For this review, take the finished solid that the model builds, in its own axes (mm). A direction names the side the tool comes from. Coordinates: 2 decimals unless noted, no trailing zeros. Write each loop counter-clockwise with the first axis right and the second up, starting at its lowest first coordinate (ties: lowest second). Pieces come first, ordered by that corner, then holes.
1) Mouldability with a two-part tool opening along Z and no side actions: class faces 1 (the face through (0, 15, -13.465)), 2 (the face through (-12.073, 24.775, -14.204)), 3 (the face through (0, 15, 13.465)), 4 (the face through (0, 16, 14.965)) as pulls with the +Z half, pulls with the -Z half, needs draft (parallel to the pull), parting line crosses it, or undercut.
2) For faces 5 (the face through (0, 1.5, 0)), 6 (the face through (0.338, 29.578, -14.226)), 7 (the face through (0, 0, 0)), list the 3-axis set-ups (+Z, -Z, +X, -X, +Y, -Y) from which the entire face can be reached by the end or side of a thin tool; tool diameter is ignored.
3) We need section B-B on x = 0. Write out the cut boundary in (y, z) (3 decimals).
4) Insertion check: P1, Ø1.5, axis at x = -2.5, z = -2.5, coming from the +Y side; P2, Ø7, axis at x = 0, y = 27, coming from the -Z side (3 decimals); P3, Ø1.9, axis at x = -7, y = 27, coming from the -Z side (3 decimals). Each pin has a flat end and moves straight along its axis. Give the tip position at first contact, or say it passes through.
5) To check wall thickness, follow line 1 along Z through (x, y) = (-12, 3.5) (3 decimals); line 2 along Y through (x, z) = (13, 8.25); line 3 along Y through (x, z) = (-7, -13.95). State the ranges of each line that lie inside material, in increasing order.
6) We need section C-C on x = -7. Write out the cut boundary in (y, z) (3 decimals).
7) We need section A-A on y = 4. Write out the cut boundary in (x, z) (3 decimals).
8) We need section D-D on y = 27. Write out the cut boundary in (x, z) (3 decimals), then the cut area to 3 significant figures.
Autodesk Inventor part; units mm, degrees
ref_plane "YZ Plane" through (0, 0, 0) normal (1, 0, 0) x (0, 1, 0)
ref_plane "XZ Plane" through (0, 0, 0) normal (0, 1, 0) x (-1, 0, 0)
ref_plane "XY Plane" through (0, 0, 0) normal (0, 0, 1) x (1, 0, 0)
sketch "Sketch1" plane through (0, 0, 0) normal (0, 1, 0) x (-1, 0, 0)
  line L0 (15, 14.965) -> (-15, 14.965)
  line L1 (-15, 14.965) -> (-15, -14.965)
  line L2 (-15, -14.965) -> (15, -14.965)
  line L3 (15, -14.965) -> (15, 14.965)
  point P0 (0, 0)
  dimension "d0" = 29.93
  dimension "d1" = 30
  dimension "d2" = 15
  dimension "d3" = 14.965
extrude "Plate1" add sketch "Sketch1" along normal blind 1.5
sketch "Sketch2" plane through (-15, 0, -13.465) normal (0, 0, -1) x (-1, 0, 0)
  line L0 (-30, 0) -> (0, 0)
  line L1 (0, 0) -> (0, 37)
  line L2 (0, 37) -> (-30, 37)
  line L3 (-30, 37) -> (-30, 0)
edge flange "Flange1" height 37 angle 90 thickness 1.5 bend radius 0.31 thickness toward (0, 0, -1) relief tear relief width 1.5 relief depth 0.75 corner gap 0.31 corner form 0 edges at (0, 1.5, -14.965) (0, 1.5, 14.965) wall of the first edge with corners at (15, 0, -13.465) (-15, 0, -13.465) (-15, 37, -13.465) (15, 37, -13.465)
bend "Bend1"
corner "Corner1"
sketch "Sketch3" plane through (-15, 37, 14.965) normal (0, 0, 1) x (1, 0, 0)
  line L0 (0, 0) -> (30, 0)
  line L1 (0, -35.19) -> (0, 0)
  circle A0 centre (15, -10) radius 10
  line L2 (0, -18.5) -> (30, -18.5)
  line L3 (30, -18.5) -> (30, -28.5)
  line L4 (30, -28.5) -> (0, -28.5)
  line L5 (0, -28.5) -> (0, -18.5)
  line L6 (30, -18.5) -> (24.0624, -5.7723)
  line L7 (0, -18.5) -> (5.9376, -5.7723)
  line L8 (0, 0) -> (30, 0)
  line L9 (30, 0) -> (30, -25)
  line L10 (30, -25) -> (0, -25)
  line L11 (0, -25) -> (0, 0)
  point P0 (15, -37)
  point P1 (15, 0)
  dimension "d15" = 10
  dimension "d16" = 0
  dimension "d17" = 20
  dimension "d18" = 8.5
  dimension "d19" = 0
  dimension "d20" = 30
  dimension "d21" = 10
  dimension "d22" = 25
extrude "Extrusion1" cut sketch "Sketch3" against normal blind 35 contours L0 A0 L7 L1 | L0 L9 L6 A0
sketch "Sketch4" plane through (15, 1.81, -14.965) normal (0, 0, -1) x (-1, 0, 0)
  arc A0 (24.0624, 29.4177) -> (5.9376, 29.4177) centre (15, 25.19) ccw
  circle A1 centre (15, 25.19) radius 2.6
  circle A2 centre (8, 25.19) radius 1.05
  circle A3 centre (22, 25.19) radius 1.05
  circle A4 centre (15, 32.19) radius 1.05
  circle A5 centre (15, 18.19) radius 1.05
  point P0 (15, -1.81)
  dimension "d25" = 5.2
  dimension "d26" = 0
  dimension "d27" = 7
  dimension "d28" = 2.1
  dimension "d29" = 7
  dimension "d30" = 0
  dimension "d31" = 2.1
  dimension "d32" = 0
  dimension "d33" = 7
  dimension "d34" = 2.1
  dimension "d35" = 7
  dimension "d36" = 0
  dimension "d37" = 2.1
extrude "Extrusion2" cut sketch "Sketch4" against normal blind 1.5
sketch "Sketch5" plane through (-15, 1.81, 14.965) normal (0, 0, 1) x (1, 0, 0)
  arc A0 (24.0624, 29.4177) -> (5.9376, 29.4177) centre (15, 25.19) ccw
  circle A1 centre (15, 25.19) radius 2.55
  point P0 (15, -1.81)
  dimension "d40" = 5.1
extrude "Extrusion3" cut sketch "Sketch5" against normal blind 1.5
equation "\"d4\" = Thickness"
equation "\"d5\" = BendReliefWidth"
equation "\"d6\" = BendReliefDepth"
equation "\"d7\" = MinimumRemnant"
equation "\"d8\" = TransitionRadius"
equation "\"d11\" = BendRadius"
equation "\"d12\" = CornerReliefSize"
equation "\"d13\" = GapSize"
equation "\"d14\" = JacobiRadiusSize"
equation "\"BendReliefWidth\" = Thickness"
equation "\"BendReliefDepth\" = 0.5 * Thickness"
equation "\"CornerReliefSize\" = 4 * Thickness"
equation "\"MinimumRemnant\" = 2 * Thickness"
equation "\"TransitionRadius\" = BendRadius"
equation "\"JacobiRadiusSize\" = BendRadius"
equation "\"GapSize\" = Thickness"
properties part number "partpart" material "Aluminum 6061-AHC"
Result:
1. face 1: undercut
1. face 2: needs draft
1. face 3: undercut
1. face 4: pulls with the +Z half
2. face 5: +X, -X, +Y
2. face 6: -Z
2. face 7: +Z, -Z, +X, -X, -Y
3. outline: (0, -13.155) arc R1.81 ccw to (1.81, -14.965) - (18.95, -14.965) - (18.95, -13.465) - (1.81, -13.465) arc R0.31 cw to (1.5, -13.155) - (1.5, 13.155) arc R0.31 cw to (1.81, 13.465) - (24.45, 13.465) - (24.45, 14.965) - (1.81, 14.965) arc R1.81 ccw to (0, 13.155) - close; (21.05, -14.965) - (24.4, -14.965) - (24.4, -13.465) - (21.05, -13.465) - close; (29.55, 13.465) - (37, 13.465) - (37, 14.965) - (29.55, 14.965) - close; (29.6, -14.965) - (32.95, -14.965) - (32.95, -13.465) - (29.6, -13.465) - close; (35.05, -14.965) - (37, -14.965) - (37, -13.465) - (35.05, -13.465) - close
4. P1: stops at y = 1.5
4. P2: stops at z = -14.965
4. P3: stops at z = 13.465
5. line 1: z = -14.965 to -13.465, 13.465 to 14.965
5. line 2: y = 0 to 1.5
5. line 3: y = 0.18 to 25.95, 28.05 to 34.14
6. outline: (0, -13.155) arc R1.81 ccw to (1.81, -14.965) - (25.95, -14.965) - (25.95, -13.465) - (1.81, -13.465) arc R0.31 cw to (1.5, -13.155) - (1.5, 13.155) arc R0.31 cw to (1.81, 13.465) - (34.141, 13.465) - (34.141, 14.965) - (1.81, 14.965) arc R1.81 ccw to (0, 13.155) - close; (28.05, -14.965) - (34.141, -14.965) - (34.141, -13.465) - (28.05, -13.465) - close
7. outline: (-15, -14.965) - (15, -14.965) - (15, -13.465) - (-15, -13.465) - close; (-15, 13.465) - (15, 13.465) - (15, 14.965) - (-15, 14.965) - close
8. outline: (-11.035, -14.965) - (-8.05, -14.965) - (-8.05, -13.465) - (-11.035, -13.465) - close; (-11.035, 13.465) - (-2.55, 13.465) - (-2.55, 14.965) - (-11.035, 14.965) - close; (-5.95, -14.965) - (-2.6, -14.965) - (-2.6, -13.465) - (-5.95, -13.465) - close; (2.55, 13.465) - (11.035, 13.465) - (11.035, 14.965) - (2.55, 14.965) - close; (2.6, -14.965) - (5.95, -14.965) - (5.95, -13.465) - (2.6, -13.465) - close; (8.05, -14.965) - (11.035, -14.965) - (11.035, -13.465) - (8.05, -13.465) - close
8. area: 44.5 mm2
